from build123d import *

# Parameters (mm, degrees)
CYLINDER002_R     = 20
CYLINDER002_DEPTH = 20
CYLINDER001_R     = 1.35
CYLINDER001_DEPTH = 10
ARRAY001_COUNT    = 3
CYLINDER_R        = 4.1
CYLINDER_DEPTH    = 2.25
SKETCH002_W       = 5
SKETCH002_H       = 4.7
ARRAY_Z_COUNT     = 6
ARRAY_Z_PITCH     = 1.6


with BuildPart() as clone_of_upperdomain:
    # Cylinder002 → Cylinder002 (new body)
    with BuildSketch(Plane.XY.offset(1.25)):
        Circle(CYLINDER002_R)
    extrude(amount=CYLINDER002_DEPTH)


with BuildPart() as obj1:
    # Cylinder001 → Cylinder001 (new body)
    with BuildSketch(Plane(origin=(0, 6, -4), x_dir=(1, 0, 0), z_dir=(0, 0, 1))):
        Circle(CYLINDER001_R)
    extrude(amount=CYLINDER001_DEPTH)

    # Array001: obj1 ×3 about axis
    array001_axis = Axis((0, 0, 0), (0, 0, 1))


with BuildPart() as obj1_1:
    add(obj1.part)
    for i in range(1, ARRAY001_COUNT):
        add(obj1.part.rotate(array001_axis, i * 360 / ARRAY001_COUNT))


with BuildPart() as lensfit:
    # Cylinder → Cylinder (new body)
    with BuildSketch(Plane.XY.offset(-1)):
        Circle(CYLINDER_R)
    extrude(amount=CYLINDER_DEPTH)


with BuildPart() as obj2:
    # Sketch002 → Revolution002 (revolve)
    with BuildSketch(Plane.XZ):
        with Locations((7.5, 0.85)):
            Rectangle(SKETCH002_W, SKETCH002_H)
    revolve(axis=Axis((0, 0, 0), (0, 0, 1)))


with BuildPart() as innergroovetool:
    # Sketch001 → Revolution001 (revolve)
    with BuildSketch(Plane.XZ):
        Polygon((4, 3.2), (4, 1.6), (8, 1.6), (8.8, 2.4), (8, 3.2), align=None)
    revolve(axis=Axis((0, 0, 0), (0, 0, 1)))

    # Array Z: InnerGrooveTool ×6


with BuildPart() as innergroovetool_1:
    add(innergroovetool.part)
    with Locations(*[(0, 0, -i * ARRAY_Z_PITCH) for i in range(1, ARRAY_Z_COUNT)]):
        add(innergroovetool.part)

    # Common: intersect obj2
    add(obj2.part, mode=Mode.INTERSECT)


with BuildPart() as adaptor:
    # Sketch → Revolution (revolve)
    with BuildSketch(Plane.XZ):
        Polygon((1.25, 4), (1.25, -1.5), (8, -1.5), (8, 3.2), (5, 3.2), (5, 4), align=None)
    revolve(axis=Axis((0, 0, 0), (0, 0, 1)))

    # Fusion001: union InnerGrooveTool
    add(innergroovetool_1.part)

    # Cut: cut LensFit
    add(lensfit.part, mode=Mode.SUBTRACT)

    # Cut001: cut obj1
    add(obj1_1.part, mode=Mode.SUBTRACT)

    # Cut002: cut Clone of UpperDomain
    add(clone_of_upperdomain.part, mode=Mode.SUBTRACT)


solid = adaptor.part
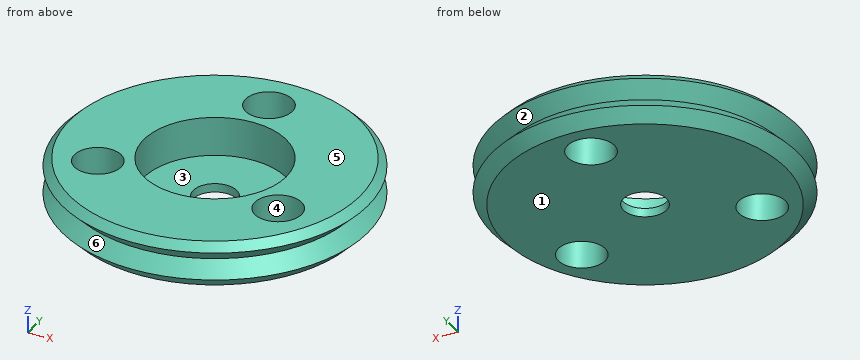
The model under review builds one solid part; all positions refer to its coordinate system, in mm. Face numbers are marked on the shaded views. A direction names the side the tool comes from. Coordinates: 2 decimals unless noted, no trailing zeros. Write each loop counter-clockwise with the first axis right and the second up, starting at its lowest first coordinate (ties: lowest second). Pieces come first, ordered by that corner, then holes. Notation, with made-up numbers: (70.5, -21.5) - (90.5, -21.5) arc R10 ccw to (90.5, -15.5) - close; hole circle Ø8 at (54.25, 7). An arc over 180 degrees is marked (long way). Answer as a JSON object with one key per item and string values. Group by question number.
1. Clearance check with flat-ended pins moving along their axes: pin 1 Ø4 at (x, y) = (0, 0) entering from -Z; pin 2 Ø2 at (x, y) = (5.2, -3) entering from +Z; pin 3 Ø1.5 at (y, z) = (-3, -1) entering from +X; pin 4 Ø2 at (x, y) = (-2, 1.5) entering from +Z. State where each tip first meets the part, or that it passes through.
2. Mouldability with a two-part tool opening along Y and no side actions: class the marked faces 4, 5 and 6 as pulls with the +Y half, pulls with the -Y half, needs draft (parallel to the pull), parting line crosses it, or undercut.
3. Add section B-B (x = 0). Give the boundary of the cut face in (y, z).
4. Add section C-C (y = -3). Give the number of separate pieces and of enclosed holes in the cut face, plus the area to 3 significant figures.
5. Add section A-A (y = 0). Give the boundary of the cut face in (x, z).
6. To check wall thickness, follow probe 1 along Y at (x, z) = (1, -1.25); probe 2 along Y at (x, z) = (-0.5, -0.95); probe 3 along X at (y, z) = (3, 0.3). State the ranges of each line that lie inside material, in increasing order.
7. Machinability: for the marked faces 1, 2 and 3, which of the approach directions +Z, -Z, +X, -X, +Y, -Y give a long, thin tool a straight path to every point of the face, cutting with its end or side? Answer none if there is none.
Findings:
{
 "1": {"pin 1": "z = -1.5", "pin 2": "through", "pin 3": "x = 8.5", "pin 4": "z = -1"},
 "2": {"face 4": "undercut", "face 5": "needs draft", "face 6": "parting line crosses it"},
 "3": {"outline": "(-8.8, -0.8) - (-8.1, -1.5) - (-1.25, -1.5) - (-1.25, -1) - (-4.1, -1) - (-4.1, 1.25) - (-8.35, 1.25) - (-8.8, 0.8) - (-8, 0) - close; (1.25, -1.5) - (4.65, -1.5) - (4.65, 1.25) - (4.1, 1.25) - (4.1, -1) - (1.25, -1) - close; (7.35, -1.5) - (8.1, -1.5) - (8.8, -0.8) - (8, 0) - (8.8, 0.8) - (8.35, 1.25) - (7.35, 1.25) - close"},
 "4": {"separate pieces": "3", "enclosed holes": "0", "area": "16.0 mm²"},
 "5": {"outline": "(-8.8, -0.8) - (-8.1, -1.5) - (-1.25, -1.5) - (-1.25, -1) - (-4.1, -1) - (-4.1, 1.25) - (-8.35, 1.25) - (-8.8, 0.8) - (-8, 0) - close; (1.25, -1.5) - (8.1, -1.5) - (8.8, -0.8) - (8, 0) - (8.8, 0.8) - (8.35, 1.25) - (4.1, 1.25) - (4.1, -1) - (1.25, -1) - close"},
 "6": {"probe 1": "-8.29 to -0.75, 0.75 to 5.09, 6.91 to 8.29", "probe 2": "-8.64 to -4.07, 4.07 to 4.75, 7.25 to 8.64", "probe 3": "-7.74 to -2.79, 2.79 to 7.74"},
 "7": {"face 1": "-Z, +X, -X, +Y, -Y", "face 2": "none", "face 3": "+Z"}
}
